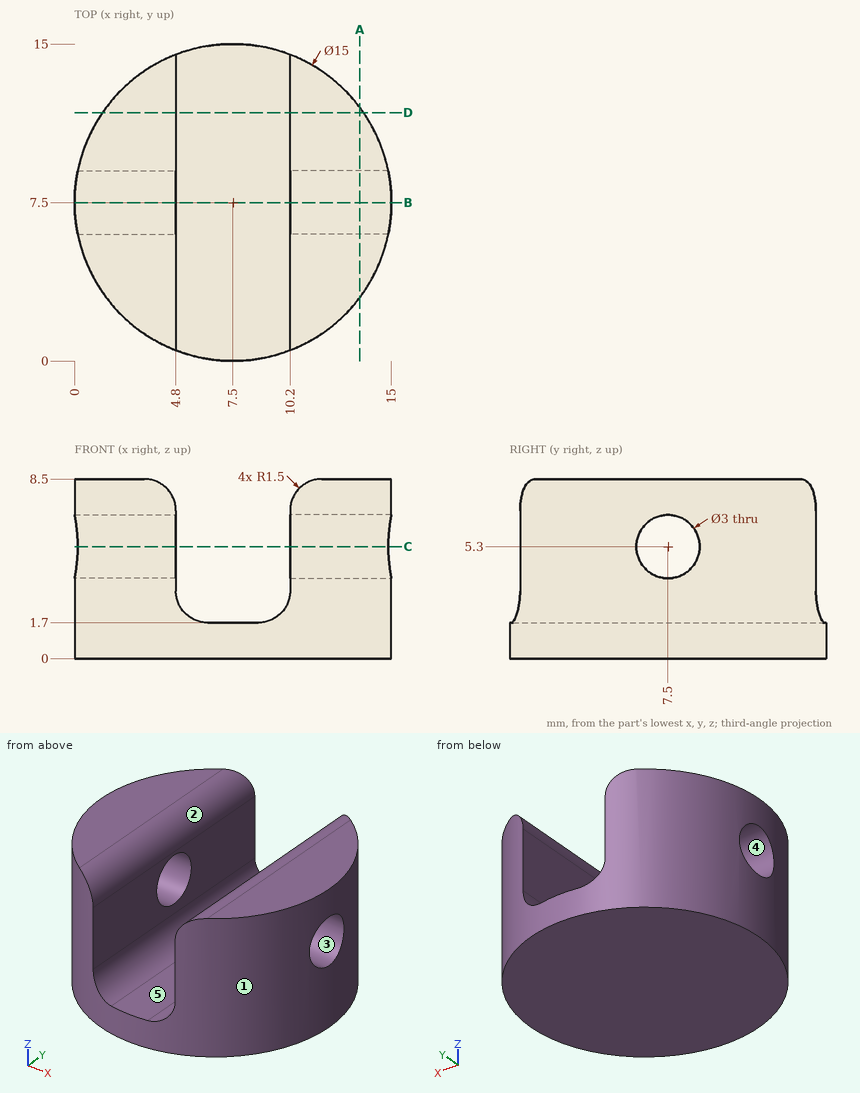
Drawing for the job (mm, zero at the part's lowest x, y, z). A direction names the side the tool comes from. Give positions to 0.01 mm unless a question says otherwise; leave off trailing zeros. Order: outer loops, then holes, each group sorted by start corner. A loop starts at its lowest first (then second) coordinate and runs counter-clockwise, first axis right, second up. Notation, with made-up numbers: M 70.5,-1.5 L 85.5,-1.5 A31 cw 85.5,33.5 Z; hole C -2,-33.5 d7. An arc over 180 degrees is marked long. Use a Markdown table: item, result. Add a question column.
(1) Probe line 1 along X through (y, z) = (13.5, 3); line 2 along X through (y, z) = (5.75, 5.25); line 3 along Z through (x, y) = (7.75, 3.25). List the from-to ranges inside material, lowest first. Write a range as [from, to].
(2) Saw through at A-A, the plane x = 13.5. Give the cut face in (y, z).
(3) Saw through at D-D, the plane y = 11.75. Give the cut face in (x, z).
(4) Mould opens along Y. For the marked faces 1, 2 and 3 say: +Y half, -Y half, draft (parallel to the pull), parting line (faces both ways), or undercut.
(5) Saw through at B-B, the plane y = 7.5. Give the cut face in (x, z), and give its area (3 significant figures).
(6) 3-axis set-ups, long thin cutter, end or side, ignore diameter. For the marked faces 4 and 5: which of +Z, -Z, +X, -X, +Y, -Y reach the whole face in a straight line?
(7) Saw through at C-C, the plane z = 5.3. Give the cut face in (x, y), and give its area (3 significant figures).
(8) Drop flat-ended pins along their axis: P1, Ø2, axis at x = 2.5, z = 1.5, coming from the -Y side; P2, Ø5, axis at y = 4, z = 1.5, coming from the +X side; P3, Ø1.9, axis at y = 5, z = 5.5, coming from the -X side. Give the stop position or say it passes through.
Answer key:
| question | item | result |
|---|---|---|
| 1 | line 1 | [3, 4.81], [10.19, 12] |
| 1 | line 2 | [0.21, 4.8], [10.2, 14.79] |
| 1 | line 3 | [0, 1.7] |
| 2 | outline | M 3,0 L 12,0 L 12,8.5 L 3,8.5 Z; hole C 7.5,5.3 d3 |
| 3 | outline | M 1.32,0 L 13.68,0 L 13.68,8.5 L 11.7,8.5 A1.5 ccw 10.2,7 L 10.2,3.2 A1.5 cw 8.7,1.7 L 6.3,1.7 A1.5 cw 4.8,3.2 L 4.8,7 A1.5 ccw 3.3,8.5 L 1.32,8.5 Z |
| 4 | face 1 | parting line |
| 4 | face 2 | draft |
| 4 | face 3 | undercut |
| 5 | outline | M 0,0 L 15,0 L 15,3.8 L 10.2,3.8 L 10.2,3.2 A1.5 cw 8.7,1.7 L 6.3,1.7 A1.5 cw 4.8,3.2 L 4.8,3.8 L 0,3.8 Z; M 0,6.8 L 4.8,6.8 L 4.8,7 A1.5 ccw 3.3,8.5 L 0,8.5 Z; M 10.2,6.8 L 15,6.8 L 15,8.5 L 11.7,8.5 A1.5 ccw 10.2,7 Z |
| 5 | area | 62.0 mm^2 |
| 6 | face 4 | +X, -X |
| 6 | face 5 | +Z, +Y, -Y |
| 7 | outline | M 0.15,6 A7.5 ccw 4.8,0.5 L 4.8,6 Z; M 0.15,9 L 4.8,9 L 4.8,14.5 A7.5 ccw Z; M 10.2,0.5 A7.5 ccw 14.85,6 L 10.2,6 Z; M 10.2,9 L 14.85,9 A7.5 ccw 10.2,14.5 Z |
| 7 | area | 69.0 mm^2 |
| 8 | P1 | y = 1.16 |
| 8 | P2 | x = 14.93 |
| 8 | P3 | x = 0.16 |
